For this review, take the finished solid that the model builds, in its own axes (mm). Face numbers are marked on the shaded views. A direction names the side the tool comes from. Coordinates: 2 decimals unless noted, no trailing zeros. Loops run counter-clockwise (first coordinate to the right, second up) from the corner with the lowest first, then second, coordinate; pieces in that order, holes last.
```python
from build123d import *

# Parameters (mm, degrees)
SKETCH1_W           = 98
SKETCH1_H           = 12
BOSS_EXTRUDE1_DEPTH = 2
SKETCH2_W           = 2
SKETCH2_H           = 12
BOSS_EXTRUDE2_DEPTH = 56
SKETCH3_R           = 1.5
CUT_EXTRUDE1_DEPTH  = 114.507708989
FILLET1_R           = 8
SKETCH4_R           = 1.5
CUT_EXTRUDE2_DEPTH  = 113.584591032


with BuildPart() as part:
    # Sketch1 → Boss-Extrude1 (new body)
    with BuildSketch(Plane(origin=(0, 0, 0), x_dir=(1, 0, 0), z_dir=(0, 1, 0))):
        with Locations((49, 6)):
            Rectangle(SKETCH1_W, SKETCH1_H)
    extrude(amount=BOSS_EXTRUDE1_DEPTH)

    # Sketch2 → Boss-Extrude2 (add)
    with BuildSketch(Plane(origin=(0, 2, 0), x_dir=(1, 0, 0), z_dir=(0, 1, 0))):
        with Locations((97, 6)):
            Rectangle(SKETCH2_W, SKETCH2_H)
    extrude(amount=BOSS_EXTRUDE2_DEPTH)

    # Sketch3 → Cut-Extrude1 (cut, through all)
    with BuildSketch(Plane(origin=(0, 2, 0), x_dir=(1, 0, 0), z_dir=(0, 1, 0))):
        with Locations(Location((6, 6, 0), (0, 0, 270))):
            Circle(SKETCH3_R)
        with Locations(Location((65, 6, 0), (0, 0, 270))):
            Circle(SKETCH3_R)
    extrude(amount=-CUT_EXTRUDE1_DEPTH, mode=Mode.SUBTRACT)

    # Fillet1
    # the kernel refuses this fillet: 8 mm, written as the material it takes off along each edge
    with BuildSketch(Plane(origin=(0, -20, 0), x_dir=(1, 0, 0), z_dir=(0, 1, 0)), Plane(origin=(0, -20, -12), x_dir=(0, 0, 1), z_dir=(0, 1, 0))) as fillet1_piece_1:
        with BuildLine():
            CenterArc((FILLET1_R, FILLET1_R), FILLET1_R, 180, 90)
            Line((0, FILLET1_R), (0, 0))
            Line((0, 0), (FILLET1_R, 0))
        make_face()
    extrude(amount=42, mode=Mode.SUBTRACT)

    # Sketch4 → Cut-Extrude2 (cut, through all)
    with BuildSketch(Plane.ZY.offset(-96)):
        with Locations((-6, 8)):
            Circle(SKETCH4_R)
        with Locations((-6, 52)):
            Circle(SKETCH4_R)
    extrude(amount=-CUT_EXTRUDE2_DEPTH, mode=Mode.SUBTRACT)


solid = part.part
```
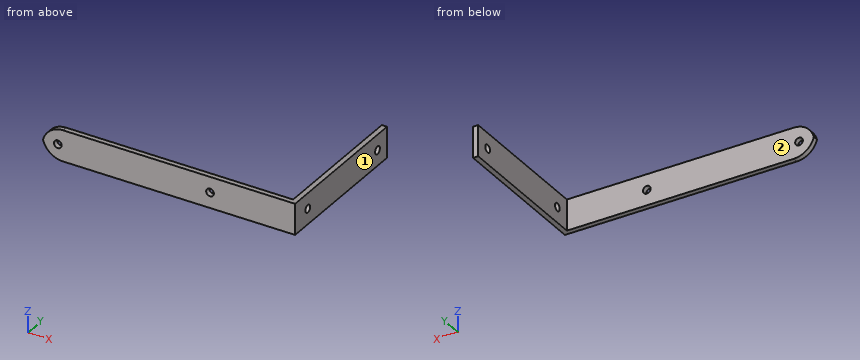
Q1. Consider section D-D (y = 27.5). State the section outline as (x, z) points.
Q2. Machinability: for the marked faces 1 and 2, which of the approach directions +Z, -Z, +X, -X, +Y, -Y give a long, thin tool a straight path to every point of the face, cutting with its end or side? Answer none if there is none.
Q3. Consider section C-C (z = -9.5). State the section outline as (x, y) points, then the cut area to 3 significant figures.
Q4. Consider section A-A (x = 65). State the section outline as (y, z) points, then the cut area to 3 significant figures.
Q5. Wall thickness on probe 1 along Y at (x, z) = (97.5, -6); probe 2 along X at (y, z) = (1.45, -6); probe 3 along X at (y, z) = (38.5, -6.75): over which ranges is each line inside the solid? List them lowest first.
Q6. For pin 1 Ø4 at (x, z) = (34.5, -1.5) entering from +Y; pin 2 Ø6 at (y, z) = (37, -1.5) entering from -X; pin 3 Ø1.8 at (x, z) = (65, -6) entering from +Y; pin 4 Ø4 at (y, z) = (52, -6) entering from +X, all flat-tipped, find the tip position at first contact; note any pin that passes through.
Q7. Consider section B-B (y = 52). State the section outline as (x, z) points, then the cut area to 3 significant figures.
Model answer:
1. outline: (96, -12) - (98, -12) - (98, 0) - (96, 0) - close
2. face 1: +Z, -Z, +X, +Y, -Y
2. face 2: +Z, -Z, -X, +Y
3. outline: (2.19, 0) - (98, 0) - (98, 58) - (96, 58) - (96, 2) - (2.19, 2) - close
3. area: 304 mm2
4. outline: (0, -12) - (2, -12) - (2, -7.5) - (0, -7.5) - close; (0, -4.5) - (2, -4.5) - (2, 0) - (0, 0) - close
4. area: 18.0 mm2
5. probe 1: y = 0 to 6.5, 9.5 to 50.5, 53.5 to 58
5. probe 2: x = 0.25 to 4.5, 7.5 to 63.5, 66.5 to 98
5. probe 3: x = 96 to 98
6. pin 1: stops at y = 2
6. pin 2: stops at x = 96
6. pin 3: passes through
6. pin 4: stops at x = 98
7. outline: (96, -12) - (98, -12) - (98, -7.5) - (96, -7.5) - close; (96, -4.5) - (98, -4.5) - (98, 0) - (96, 0) - close
7. area: 18.0 mm2
